from build123d import *

# Parameters (mm, degrees)
F0_W     = 7
F0_H     = 7
F0_R     = 1.15
F1_DEPTH = 4.5
F2_W     = 7
F2_H     = 1.5
F3_DEPTH = 10


with BuildPart() as f1:
    # F0 (on Top) → F1 (new body, symmetric)
    with BuildSketch(Plane.XY):
        Rectangle(F0_W, F0_H)
        Circle(F0_R, mode=Mode.SUBTRACT)
    extrude(amount=F1_DEPTH, both=True)

    # F2 (on face) → F3 (join)
    with BuildSketch(Plane.YZ.offset(3.5)):
        with Locations((0, -3.75)):
            Rectangle(F2_W, F2_H)
    extrude(amount=F3_DEPTH)


solid = f1.part
Design review of the part built by this model. Coordinates are the model's own, in mm. A direction names the side the tool comes from. Coordinates: 2 decimals unless noted, no trailing zeros. Order: outer loops, then holes, each group sorted by start corner. A loop starts at its lowest first (then second) coordinate and runs counter-clockwise, first axis right, second up.
Item 1: Take a section at C-C, the plane x = 3.75. Write out the cut boundary in (y, z).
Item 2: For line 1 (Y direction, x = 0, z = -1.25); line 2 (Z direction, x = 12.25, y = -1.75); line 3 (X direction, y = 3.25, z = 1.75), list the stretches that pass through material, from the lowest coordinate up.
Item 3: The part is to be moulded in two halves that separate along X. For faces 1 (the cylindrical face through (-0.91, -0.7, -0.06)), 2 (the flat face through (3.5, 0, 1)), 3 (the flat face through (1, 3.5, -1)), say which applies: pulls with the +X half, pulls with the -X half, needs draft (parallel to the pull), parting line crosses it, or undercut.
Item 4: For pin 1 Ø2 at (y, z) = (-1, 0) entering from +X; pin 2 Ø1.5 at (x, y) = (11, -0.5) entering from +Z; pin 3 Ø3 at (x, z) = (4.5, -2.5) entering from +Y, all flat-tipped, find the tip position at first contact; note any pin that passes through.
Item 5: Take a section at A-A, the plane z = 0.5. Write out the cut boundary in (x, y), then the cut area to 3 significant figures.
Item 6: For faces 4 (the flat face through (8, 0, -3)), 5 (the flat face through (-1, 1, 4.5)), list the 3-axis set-ups (+Z, -Z, +X, -X, +Y, -Y) from which the entire face can be reached by the end or side of a thin tool; tool diameter is ignored.
Item 7: Take a section at B-B, the plane x = 0. Write out the cut boundary in (y, z).
The answers:
1. outline: (-3.5, -4.5) - (3.5, -4.5) - (3.5, -3) - (-3.5, -3) - close
2. line 1: y = -3.5 to -1.15, 1.15 to 3.5
2. line 2: z = -4.5 to -3
2. line 3: x = -3.5 to 3.5
3. face 1: undercut
3. face 2: pulls with the +X half
3. face 3: needs draft
4. pin 1: stops at x = 3.5
4. pin 2: stops at z = -3
4. pin 3: stops at y = 3.5
5. outline: (-3.5, -3.5) - (3.5, -3.5) - (3.5, 3.5) - (-3.5, 3.5) - close; hole circle Ø2.3 at (0, 0)
5. area: 44.8 mm2
6. face 4: +Z, +X, +Y, -Y
6. face 5: +Z, +X, -X, +Y, -Y
7. outline: (-3.5, -4.5) - (-1.15, -4.5) - (-1.15, 4.5) - (-3.5, 4.5) - close; (1.15, -4.5) - (3.5, -4.5) - (3.5, 4.5) - (1.15, 4.5) - close
